Geometry check sheet. Reference: the model listing, model coordinates, mm. Coordinates: 2 decimals unless noted, no trailing zeros. Loops run counter-clockwise (first coordinate to the right, second up) from the corner with the lowest first, then second, coordinate; pieces in that order, holes last.
from build123d import *

# Parameters (mm, degrees)
EXTRUDE_1_DEPTH = 10


with BuildPart() as part:
    # 草图1 → 凸台-拉伸1 (new body)
    with BuildSketch(Plane(origin=(0, 0, 0), x_dir=(1, 0, 0), z_dir=(0, 1, 0))):
        with BuildLine():
            Line((12.17913919, -6.626220158), (54.557975845, 71.267018821))
            ThreePointArc((54.557975845, 71.267018821), (0, 163.06), (-54.557975845, 71.267018821))
            Line((-54.557975845, 71.267018821), (-12.17913919, -6.626220158))
            ThreePointArc((-12.17913919, -6.626220158), (0, -13.865), (12.17913919, -6.626220158))
        make_face()
        with BuildLine():
            ThreePointArc((52.801158075, 72.222838534), (0, 161.06), (-52.801158075, 72.222838534))
            Line((-52.801158075, 72.222838534), (-10.42232142, -5.670400446))
            ThreePointArc((-10.42232142, -5.670400446), (0, -11.865), (10.42232142, -5.670400446))
            Line((10.42232142, -5.670400446), (52.801158075, 72.222838534))
        make_face(mode=Mode.SUBTRACT)
    extrude(amount=EXTRUDE_1_DEPTH)


solid = part.part
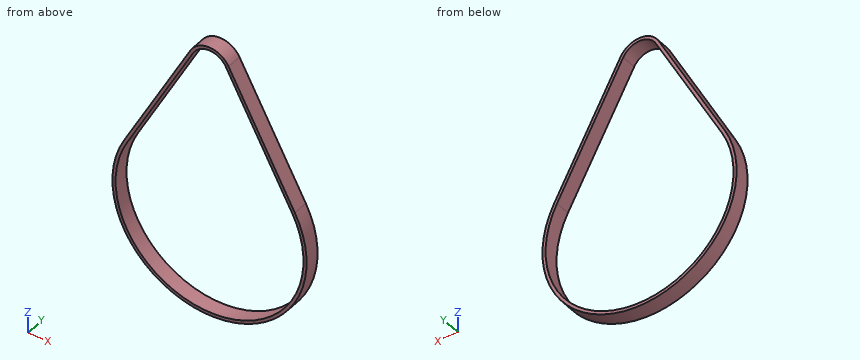
1) Depth check by flat-ended pin: pin 1 (2 mm diameter, centred on y = 4, z = -76.5, fed in from -X); pin 2 (2 mm diameter, centred on y = 8, z = -14.5, fed in from +X); pin 3 (5 mm diameter, centred on x = 29.5, y = 5, fed in from -Z). Enter the tip coordinate at first touch or a pass-through.
Data:
pin 1: stops at x = -57.51
pin 2: stops at x = 24.22
pin 3: stops at z = -156.88
2) Section check B-B on z = -100.95. Record the cut outline in (x, y), and give its area (3 significant figures).
Data:
outline: (-62.11, 0) - (-60.11, 0) - (-60.11, 10) - (-62.11, 10) - close; (60.11, 0) - (62.11, 0) - (62.11, 10) - (60.11, 10) - close
area: 40.0 mm2
3) Section check A-A on x = 0. Record the cut outline in (y, z) (3 decimals), and give its area (3 significant figures).
Data:
outline: (0, -163.06) - (10, -163.06) - (10, -161.06) - (0, -161.06) - close; (0, 11.865) - (10, 11.865) - (10, 13.865) - (0, 13.865) - close
area: 40.0 mm2
4) Section check C-C on y = 8.25. Record the cut outline in (x, z) (3 decimals).
Data:
outline: (-54.558, -71.267) arc R62.11 ccw (long way) to (54.558, -71.267) - (12.179, 6.626) arc R13.865 ccw to (-12.179, 6.626) - close; hole (-52.801, -72.223) arc R60.11 ccw (long way) to (52.801, -72.223) - (10.422, 5.67) arc R11.865 ccw to (-10.422, 5.67) - close
5) Material ranges on probe 1 along X at (y, z) = (7.5, -100.95); probe 2 along X at (y, z) = (6.75, -47.5); probe 3 along Z at (x, y) = (-30.5, 8), recorded low to high.
Data:
probe 1: x = -62.11 to -60.11, 60.11 to 62.11
probe 2: x = -41.63 to -39.35, 39.35 to 41.63
probe 3: z = -155.06 to -152.75, -31.23 to -27.05
